Here's how the part is built. I have some questions about the finished solid (model axes, mm). A direction names the side the tool comes from. Round coordinates to 2 decimals unless told otherwise and drop trailing zeros. Order: outer loops, then holes, each group sorted by start corner. A loop starts at its lowest first (then second) coordinate and runs counter-clockwise, first axis right, second up.
```python
from build123d import *

# Parameters (mm, degrees)
F1_DEPTH      = 228.6
F1_DEPTH_BACK = 228.6


with BuildPart() as f1:
    # F0 (on Right) → F1 (new body, two sides)
    with BuildSketch(Plane.YZ) as f1_sk:
        with BuildLine():
            Line((-117.475, 0), (0, 0))
            Line((0, 0), (0, 6.35))
            Line((0, 6.35), (-117.475, 6.35))
            ThreePointArc((-117.475, 6.35), (-119.720064, 7.279936), (-120.65, 9.525))
            Line((-120.65, 9.525), (-120.65, 113.160496))
            ThreePointArc((-120.65, 113.160496), (-119.275056, 115.775916), (-116.341071, 116.126104))
            Line((-116.341071, 116.126104), (203.596992, -6.205272))
            Line((203.596992, -6.205272), (205.148099, 0))
            Line((205.148099, 0), (-114.073214, 122.05732))
            ThreePointArc((-114.073214, 122.05732), (-122.875167, 121.006757), (-127, 113.160496))
            Line((-127, 113.160496), (-127, 9.525))
            ThreePointArc((-127, 9.525), (-124.210192, 2.789808), (-117.475, 0))
        make_face()
    extrude(amount=F1_DEPTH)
    extrude(f1_sk.sketch, amount=-F1_DEPTH_BACK)


solid = f1.part
```
1. I need wall thicknesses on probe 1 along Z at (x, y) = (-84, -80); probe 2 along Z at (x, y) = (-160, -111); probe 3 along Z at (x, y) = (-117, 183.5). Which ranges of each line are inside material? Lowest first, please.
Evaluation:
probe 1: z = 0 to 6.35, 102.23 to 109.03
probe 2: z = 0 to 6.35, 114.08 to 120.88
probe 3: z = 1.48 to 8.28
2. I'm going to push flat-ended pins straight in: P1, Ø4, axis at x = -120.5, y = -15.5, coming from the -Z side; P2, Ø6, axis at x = 138.5, y = 27.5, coming from the +Z side. Where does each tip first touch, or does it pass through?
Evaluation:
P1: stops at z = 0
P2: stops at z = 69.07
3. If we section it at D-D, the plane y = 99: Write out the boundary of the cut face in (x, z), and give its area (3 significant figures).
Evaluation:
outline: (-228.6, 33.79) - (228.6, 33.79) - (228.6, 40.59) - (-228.6, 40.59) - close
area: 3,110 mm2
4. On a 3-axis mill with a long thin cutter (end or side, diameter ignored), from which of +Z, -Z, +X, -X, +Y, -Y can I reach the whole of each face in a straight line? I mean faces 1 (the flat face through (-228.6, 1, 73)), 2 (the flat face through (3, -120.65, 61)), 3 (the flat face through (3, -60, 0)). Say none if no direction works.
Evaluation:
face 1: +Z, -Z, -X, +Y, -Y
face 2: +X, -X
face 3: -Z, +X, -X, -Y
5. If we section it at C-C, the plane z = 65.5: Write out the boundary of the cut face in (x, y).
Evaluation:
outline: (-228.6, -127) - (228.6, -127) - (228.6, -120.65) - (-228.6, -120.65) - close; (-228.6, 16.06) - (228.6, 16.06) - (228.6, 33.84) - (-228.6, 33.84) - close
6. If we section it at A-A, the plane y = -98.5: Write out the boundary of the cut face in (x, z), and give its area (3 significant figures).
Evaluation:
outline: (-228.6, 0) - (228.6, 0) - (228.6, 6.35) - (-228.6, 6.35) - close; (-228.6, 109.3) - (228.6, 109.3) - (228.6, 116.1) - (-228.6, 116.1) - close
area: 6,010 mm2
7. If we mould it in two halves opening along Z, with no side actions, what happens to faces 4 (the cylindrical face through (3.2, -122.77, 121.08)), 5 (the flat face through (228.6, 1, 73)), 6 (the flat face through (3.2, 41.388, 55.817))? For each: released by +Z, released by -Z, zero draft, split by the parting line, or undercut.
Evaluation:
face 4: released by +Z
face 5: zero draft
face 6: undercut
